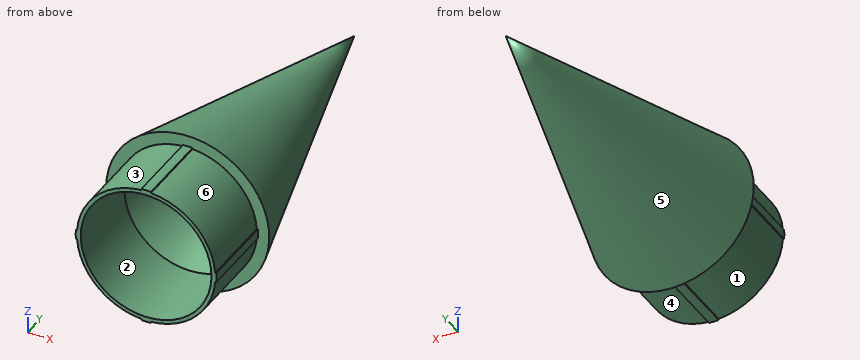
Autodesk Inventor part; units mm, degrees
ref_plane "YZ Plane" through (0, 0, 0) normal (1, 0, 0) x (0, 1, 0)
ref_plane "XZ Plane" through (0, 0, 0) normal (0, 1, 0) x (-1, 0, 0)
ref_plane "XY Plane" through (0, 0, 0) normal (0, 0, 1) x (1, 0, 0)
sketch "Sketch1" plane through (0, 0, 0) normal (1, 0, 0) x (0, 1, 0)
  line L0 (0, -22.86) -> (-25.4, -22.86)
  line L1 (-25.4, -22.86) -> (-25.4, 0)
  line L2 (-25.4, 0) -> (0, 0)
  line L3 (101.6, 0) -> (0, -26.924)
  line L4 (101.6, 0) -> (0, 0)
  line L5 (1.2682, -25.276) -> (91.8637, -1.2682)
  line L6 (-24.13, -21.59) -> (-1.27, -21.59)
  line L7 (-1.27, -21.59) -> (1.2682, -21.59)
  line L8 (-24.13, -21.59) -> (-25.4, -21.59)
  line L9 (91.8637, -1.2682) -> (96.6492, 0)
  line L10 (1.2682, -21.59) -> (1.2682, -25.276)
  line L11 (0, -26.924) -> (0, -22.86)
  dimension "d27" = 1.27
revolve "Revolution1" add sketch "Sketch1" angle 360 about axis through (0, 101.6, 0) along (0, -1, 0) contours L0 L1 L8 L6 L7 L10 L5 L9 L4 L3 L11
revolve "Revolution2" add sketch "Sketch1" angle 360 about axis through (0, -25.4, 0) along (0, 1, 0) contours L1 L2 L4 L9 L5 L10 L7 L6 L8
sketch "Sketch2" plane through (0, -25.4, 0) normal (0, -1, 0) x (1, 0, 0)
  line L0 (0, 0) -> (22.86, 0)
  circle A0 centre (0, 0) radius 22.86
  arc A1 (23.1962, -1.5875) -> (23.1962, 1.5875) centre (0, 0) ccw
  line L1 (22.8048, 1.5875) -> (23.1962, 1.5875)
  line L2 (22.8048, -1.5875) -> (23.1962, -1.5875)
  line L3 (0, -22.86) -> (1.5875, -22.86)
  line L4 (0, -22.86) -> (1.5875, -22.86) construction
  line L5 (0, -22.86) -> (-1.5875, -22.86)
  circle A2 centre (0, 0) radius 23.241
  line L6 (-1.5875, -22.8048) -> (-1.5875, -23.1867)
  line L7 (1.5875, -22.8048) -> (1.5875, -23.1867)
  line L8 (-22.86, 0) -> (-22.86, -1.5875)
  line L9 (-22.86, 0) -> (-22.86, 1.5875)
  line L10 (-22.8048, 1.5875) -> (-23.1867, 1.5875)
  line L11 (-22.8048, -1.5875) -> (-23.1867, -1.5875)
  line L12 (0, 22.86) -> (1.5875, 22.86)
  line L13 (0, 22.86) -> (1.5875, 22.86) construction
  line L14 (0, 22.86) -> (-1.5875, 22.86)
  line L15 (0, 22.86) -> (1.5875, 22.86) construction
  line L16 (-1.5875, 22.8048) -> (-1.5875, 23.1867)
  line L17 (1.5875, 22.8048) -> (1.5875, 23.1867)
  dimension "d14" = 1.5875
  dimension "d16" = 1.5875
  dimension "d17" = 0.381
  dimension "d18" = 1.5875
  dimension "d19" = 1.5875
  dimension "d21" = 1.5875
  dimension "d22" = 0
  dimension "d23" = 1.5875
  dimension "d24" = 180
extrude "Extrusion1" add sketch "Sketch2" against normal blind 25.4 contours A0 L1 A2 L2 | A0 L12 L17 | L1 A1 L2 A2 | L7 L3 A0 | L14 L16 A2 L17 L12 | A0 L16 L14 | L5 L6 A0 | L3 L7 A2 L6 L5 | A0 L9 L10 | L10 L9 L8 L11 A2 | L11 L8 A0
revolve "Revolution3" cut sketch "Sketch1" angle 360 about axis through (0, -25.4, 0) along (0, 1, 0) contours L1 L2 L4 L9 L5 L10 L7 L6 L8
revolve "Revolution4" cut sketch "Sketch1" angle 360 about axis through (0, 101.6, 0) along (0, -1, 0) contours L1 L2 L4 L9 L5 L10 L7 L6 L8
properties part number "Nose Cone MK I"
Work out the finished part from the listing and answer in its coordinate system (mm). Face numbers are marked on the shaded views. A direction names the side the tool comes from. Give positions to 0.01 mm unless a question says otherwise; leave off trailing zeros. Order: outer loops, then holes, each group sorted by start corner. A loop starts at its lowest first (then second) coordinate and runs counter-clockwise, first axis right, second up. Notation, with made-up numbers: M 16,65 L 51,65 A14 cw 51,78 Z; hole C 55,56.5 d10. An arc over 180 degrees is marked long. Return JSON: item names as keys, results as strings.
1) Section A-A, the plane y = 89 is taken. Write down the section's boundary in (x, z), plus the area to 3 significant figures.
Resolved:
{"outline": "C 0,0 d6.68; hole C 0,0 d4.05", "area": "22.1 mm^2"}
2) Straight lines are drawn through the part: line 1 along X through (y, z) = (-19, 0); line 2 along Z through (x, y) = (0, -20); line 3 along X through (y, z) = (26, 10.5). For each, find the intervals that lie inside material, in ascending order. Write a range as [from, to].
Resolved:
{"line 1": "[-23.24, -21.59], [21.59, 23.25]", "line 2": "[-23.24, -21.59], [21.59, 23.24]", "line 3": "[-17.06, -15.5], [15.5, 17.06]"}
3) A tool of negligible diameter and unlimited length cuts with its end or side. For the marked faces 4, 5 and 6, from which of +Z, -Z, +X, -X, +Y, -Y can it reach the whole face along a straight path? Write none if from no direction.
Resolved:
{"face 4": "-Z, +X, -Y", "face 5": "+Y", "face 6": "+Z, +X, -Y"}
4) For a pull along Z with two mould halves and no side action, classify the marked faces 1, 2 and 3 as +Z half, -Z half, draft (parallel to the pull), parting line (faces both ways), or undercut.
Resolved:
{"face 1": "-Z half", "face 2": "undercut", "face 3": "+Z half"}
5) Section B-B, the plane y = 67.5 is taken. Write down the section's boundary in (x, z).
Resolved:
{"outline": "C 0,0 d18.07; hole C 0,0 d15.45"}
6) Each of these flat-tipped pins is pushed along its axis until it touches: pin 1 (2 mm diameter, centred on y = 72, z = -4.5, fed in from +X); pin 2 (10 mm diameter, centred on x = -3, y = 39, fed in from -Z); pin 3 (8 mm diameter, centred on y = 7, z = -18.5, fed in from +X). Where does it stop, or does it pass through?
Resolved:
{"pin 1": "x = 7.1", "pin 2": "z = -17.79", "pin 3": "x = 20.73"}
